Read the model definition and answer for the solid it produces. Units are mm, in the model's axes. Give positions to 0.01 mm unless a question says otherwise; leave off trailing zeros. Loops run counter-clockwise (first coordinate to the right, second up) from the corner with the lowest first, then second, coordinate; pieces in that order, holes last. Notation, with made-up numbers: (-18, 52.25) - (29, 52.25) arc R13 cw to (29, 66.25) - close; hole circle Ø11 at (48, 52.5). An arc over 180 degrees is marked (long way). Use a Markdown table: item, result. Add a question column.
Item 1: For a pull along X with two mould halves and no side action, classify faces 1 (the face through (-2, 3, 5)), 2 (the face through (-1.115, 1.216, 1.676)), 3 (the face through (-0.59, -4.46, 2.47)) as +X half, -X half, draft (parallel to the pull), parting line (faces both ways), or undercut.
Item 2: Each of these flat-tipped pins is pushed along its axis until it touches: P1, Ø1.5, axis at y = -3.5, z = 2, coming from the -X side; P2, Ø1, axis at x = 1.5, z = 3.5, coming from the -Y side; P3, Ø1, axis at x = 1, z = 3, coming from the +Y side. Where does it stop, or does it pass through?
Item 3: A cutting plane is placed at C-C (z = 3.75). Determine the outline of the cut face in (x, y), plus the area to 3 significant figures.
Item 4: Consider probe 1 along Y at (x, z) = (0, 2.6); probe 2 along X at (y, z) = (1.5, 4); probe 3 along X at (y, z) = (-3.5, 1.45). Determine where each line is inside the solid, lowest interval first. Write a range as [from, to].
Item 5: A cutting plane is placed at A-A (x = 0). Determine the outline of the cut face in (y, z), plus the area to 3 significant figures.
Item 6: A cutting plane is placed at D-D (z = 4.25). Determine the outline of the cut face in (x, y).
Autodesk Fusion 360 part; units mm, degrees
sketch "Sketch1" plane through (0, 0, 0) normal (0, 0, 1) x (1, 0, 0)
  circle A0 centre (0, 0) radius 4.5
  circle A1 centre (0, 0) radius 1.5
  dimension "d1" = 9
  dimension "d4" = 3
extrude "Extrude1" add sketch "Sketch1" along normal blind 5
hole "Hole1" at (0, 0, 5) direction (0, 0, -1) diameter 3.3 depth 10 tip angle 118 countersink diameter 6.5 countersink angle 90
chamfer "Chamfer1" distance 0.5 angle 45 2 edges at (-4.1955, -1.6273, 5) (-4.1955, -1.6273, 0)
Geometry says:
| question | item | result |
|---|---|---|
| 1 | face 1 | draft |
| 1 | face 2 | undercut |
| 1 | face 3 | parting line |
| 2 | P1 | x = -3.56 |
| 2 | P2 | y = -4.39 |
| 2 | P3 | y = 4.47 |
| 3 | outline | circle Ø9 at (0, 0); hole circle Ø4 at (0, 0) |
| 3 | area | 51.1 mm² |
| 4 | probe 1 | [-4.5, -1.65], [1.65, 4.5] |
| 4 | probe 2 | [-4.24, -1.68], [1.68, 4.24] |
| 4 | probe 3 | [-2.83, 2.83] |
| 5 | outline | (-4.5, 0.5) - (-4, 0) - (-1.65, 0) - (-1.65, 3.4) - (-3.25, 5) - (-4, 5) - (-4.5, 4.5) - close; (1.65, 0) - (4, 0) - (4.5, 0.5) - (4.5, 4.5) - (4, 5) - (3.25, 5) - (1.65, 3.4) - close |
| 5 | area | 25.4 mm² |
| 6 | outline | circle Ø9 at (0, 0); hole circle Ø5 at (0, 0) |
